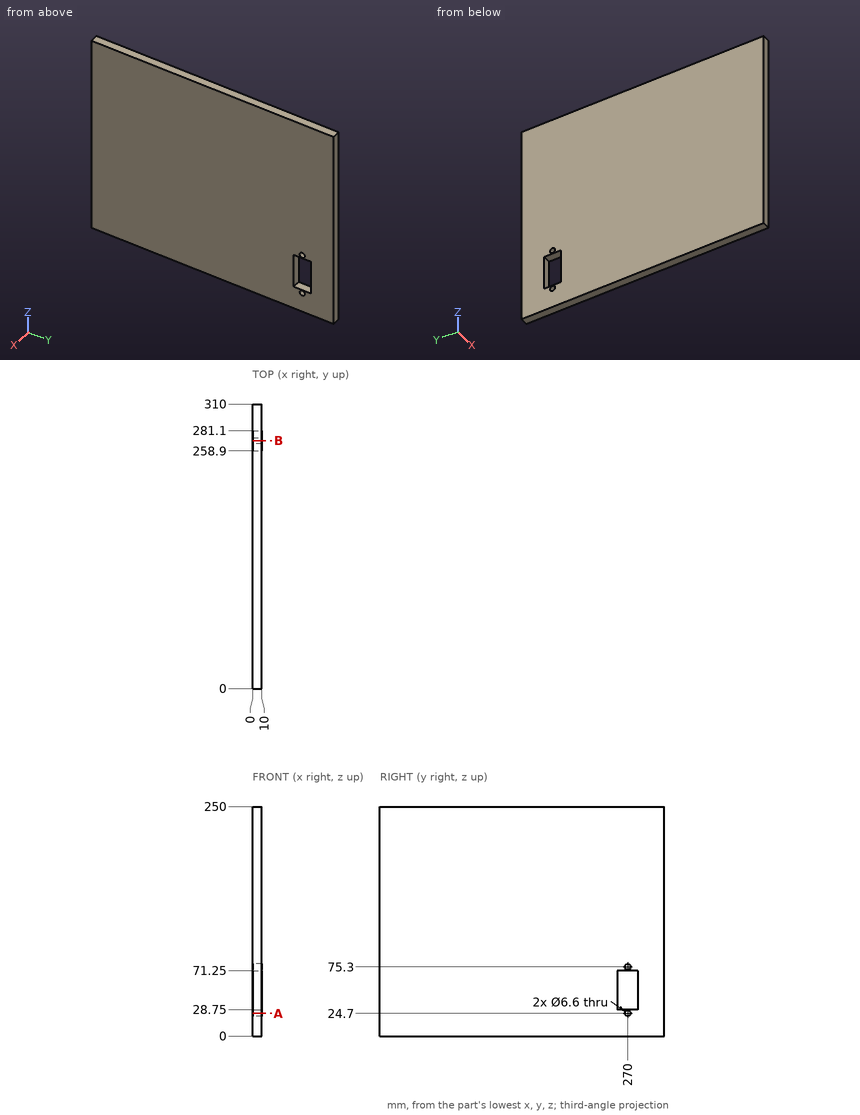
Check sheet for the drawn part. Datum: minimum x, y, z corner. Units: mm. Round coordinates to 2 decimals unless told otherwise and drop trailing zeros. Loops run counter-clockwise (first coordinate to the right, second up) from the corner with the lowest first, then second, coordinate; pieces in that order, holes last. Notation, with made-up numbers: (-31.5, 47) -> (-20.5, 47) arc R23 cw to (-20.5, 55) -> close; hole circle Ø11 at (39.25, 67). An arc over 180 degrees is marked (long way). Put each result on its own line as item: value. Start each with the question number.
1. Section check B-B (y = 270). Enter the section's corners in (x, z), plus the area to 3 significant figures.
2. Section check A-A (z = 24.7). Enter the section's corners in (x, y), plus the area to 3 significant figures.
3. Scan lines: probe 1 along Z at (x, y) = (2, 270); probe 2 along Y at (x, z) = (9.25, 25); probe 3 along Y at (x, z) = (5.5, 33). Record each from-to range of solid material in increasing order.
Findings:
1. outline: (0, 0) -> (10, 0) -> (10, 21.4) -> (0, 21.4) -> close; (0, 28) -> (10, 28) -> (10, 28.75) -> (0, 28.75) -> close; (0, 71.25) -> (10, 71.25) -> (10, 72) -> (0, 72) -> close; (0, 78.6) -> (10, 78.6) -> (10, 250) -> (0, 250) -> close
1. area: 1,940 mm^2
2. outline: (0, 0) -> (10, 0) -> (10, 266.7) -> (0, 266.7) -> close; (0, 273.3) -> (10, 273.3) -> (10, 310) -> (0, 310) -> close
2. area: 3,030 mm^2
3. probe 1: z = 0 to 21.4, 28 to 28.75, 71.25 to 72, 78.6 to 250
3. probe 2: y = 0 to 266.71, 273.29 to 310
3. probe 3: y = 0 to 258.9, 281.1 to 310
